from build123d import *

# Parameters (mm, degrees)
BOSS_EXTRUDE1_DEPTH     = 63.5
CUT_EXTRUDE1_DEPTH      = 157.189348228
CUT_EXTRUDE1_DEPTH_BACK = 38.1
CUT_EXTRUDE2_DEPTH      = 157.189348228
CUT_EXTRUDE3_DEPTH      = 180.268046511
SKETCH5_R               = 31.75
CUT_EXTRUDE4_DEPTH      = 19.05
SKETCH6_R               = 9.525
CUT_EXTRUDE5_DEPTH      = 157.189348228
SKETCH7_R               = 15.875
CUT_EXTRUDE6_DEPTH      = 148.69723254


with BuildPart() as part:
    # Sketch1 → Boss-Extrude1 (new body)
    with BuildSketch(Plane(origin=(0, 0, 0), x_dir=(1, 0, 0), z_dir=(0, 1, 0))):
        with BuildLine():
            Line((0, -50.8), (-133.35, -50.8))
            Line((-133.35, -50.8), (-133.35, 50.8))
            Line((-133.35, 50.8), (0, 50.8))
            ThreePointArc((0, 50.8), (50.8, 0), (0, -50.8))
        make_face()
    extrude(amount=BOSS_EXTRUDE1_DEPTH)

    # Sketch2 → Cut-Extrude1 (cut, two sides: drawn at the far end of the back side and taken through both)
    with BuildSketch(Plane(origin=(0, 63.5, 0), x_dir=(1, 0, 0), z_dir=(0, 1, 0)).offset(-CUT_EXTRUDE1_DEPTH_BACK)):
        Polygon((-31.75, 348.168195874), (-31.75, 50.8), (-31.75, -50.8), (-31.75, -348.168195874), (562.986391748, -348.168195874), (562.986391748, 348.168195874), align=None)
    extrude(amount=CUT_EXTRUDE1_DEPTH + CUT_EXTRUDE1_DEPTH_BACK, mode=Mode.SUBTRACT)

    # Sketch3 → Cut-Extrude2 (cut, through all)
    with BuildSketch(Plane(origin=(0, 63.5, 0), x_dir=(1, 0, 0), z_dir=(0, 1, 0))):
        Polygon((-133.35, -50.8), (-50.8, -50.8), (-133.35, -3.139735278), align=None)
    extrude(amount=-CUT_EXTRUDE2_DEPTH, mode=Mode.SUBTRACT)

    # Sketch4 → Cut-Extrude3 (cut, through all)
    with BuildSketch(Plane(origin=(0, 0, -50.8), x_dir=(-1, 0, 0), z_dir=(0, 0, -1))):
        Polygon((133.35, 63.5), (107.95, 63.5), (133.35, 38.1), align=None)
    extrude(amount=-CUT_EXTRUDE3_DEPTH, mode=Mode.SUBTRACT)

    # Sketch5 → Cut-Extrude4 (cut)
    with BuildSketch(Plane(origin=(0, 63.5, 0), x_dir=(1, 0, 0), z_dir=(0, 1, 0))):
        with Locations((-31.75, 0)):
            Circle(SKETCH5_R)
    extrude(amount=-CUT_EXTRUDE4_DEPTH, mode=Mode.SUBTRACT)

    # Sketch6 → Cut-Extrude5 (cut, through all)
    with BuildSketch(Plane(origin=(0, 63.5, 0), x_dir=(1, 0, 0), z_dir=(0, 1, 0))):
        with Locations(Location((-82.55, 25.4, 0), (0, 0, 270))):
            Circle(SKETCH6_R)
    extrude(amount=-CUT_EXTRUDE5_DEPTH, mode=Mode.SUBTRACT)

    # Sketch7 → Cut-Extrude6 (cut, through all)
    with BuildSketch(Plane(origin=(0, 25.4, 0), x_dir=(1, 0, 0), z_dir=(0, 1, 0))):
        with Locations(Location((0, 0, 0), (0, 0, 270))):
            Circle(SKETCH7_R)
    extrude(amount=-CUT_EXTRUDE6_DEPTH, mode=Mode.SUBTRACT)


solid = part.part
Part model, mm, in its own coordinate system. A direction names the side the tool comes from. Give positions to 0.01 mm unless a question says otherwise; leave off trailing zeros. Loops run counter-clockwise (first coordinate to the right, second up) from the corner with the lowest first, then second, coordinate; pieces in that order, holes last. Notation, with made-up numbers: (4.25, 40.25) -> (46.25, 40.25) arc R5 cw to (46.25, 46.25) -> close; hole circle Ø1 at (47.25, 37.25). An arc over 180 degrees is marked (long way). Write each question's results on one line, items separated by ' | '. Start each with the question number.
Q1. Wall check: L1, parallel to X at y = 8, z = 0 (3 decimals); L2, parallel to Y at x = -26.5, z = 26.5; L3, parallel to X at y = 5.5, z = -9.5. Give the ranges that are in metal, low to high.
Q2. Pull direction Z, two halves, no side cores. Call faces 1 (the face through (-91.5, 32.2, 27.3)), 2 (the face through (-15.497, 12.878, -3.441)), 3 (the face through (18, 25.4, -1)), 4 (the face through (-63.492, 54.108, -0.698)): +Z half, -Z half, draft (parallel to the pull), parting line (faces both ways), or undercut.
Q3. Band-saw the part on C-C on y = 35. List the corners of the cut face in (x, z) (3 decimals).
Q4. Band-saw the part on D-D on x = -82.55. List the corners of the cut face in (y, z) (3 decimals).
Q5. Band-saw the part on B-B on y = 22. List the corners of the cut face in (x, z) (3 decimals).
Q6. Pin check, flat tips, straight feed: P1, Ø25, axis at x = 29.5, z = 15, coming from the +Y side; P2, Ø10, axis at y = 9, z = 40.5, coming from the +X side; P3, Ø1, axis at x = 30.5, y = 21, coming from the +Z side; P4, Ø10, axis at x = -87.5, z = -39.5, coming from the -Y side. Stop position of each tip, or through.
Q7. Band-saw the part on A-A on z = 0. List the corners of the cut face in (x, y) (3 decimals).
Q8. Which spindle directions (+Z, -Z, +X, -X, +Y, -Y) get a long thin tool onto all of the face, cutting with end or side? Do faces 5 (the face through (-44, 44.45, 0)), 6 (the face through (-31.75, 40, -1)), 7 (the face through (-69, 63.5, -12)). Say none if no direction does.
Results are:
1) L1: x = -133.35 to -15.875, 15.875 to 50.8 | L2: y = 0 to 25.4 | L3: x = -133.35 to -12.72, 12.72 to 49.9
2) face 1: +Z half | face 2: undercut | face 3: draft | face 4: undercut
3) outline: (-133.35, -50.8) -> (-31.75, -50.8) -> (-31.75, 50.8) -> (-50.8, 50.8) -> (-133.35, 3.14) -> close; hole circle Ø19.05 at (-82.55, -25.4)
4) outline: (0, -50.8) -> (63.5, -50.8) -> (63.5, -34.925) -> (0, -34.925) -> close; (0, -15.875) -> (63.5, -15.875) -> (63.5, 32.469) -> (0, 32.469) -> close
5) outline: (-133.35, -50.8) -> (0, -50.8) arc R50.8 ccw to (0, 50.8) -> (-50.8, 50.8) -> (-133.35, 3.14) -> close; hole circle Ø19.05 at (-82.55, -25.4); hole circle Ø31.75 at (0, 0)
6) P1: stops at y = 25.4 | P2: stops at x = 36.34 | P3: stops at z = 41 | P4: stops at y = 0
7) outline: (-133.35, 0) -> (-15.875, 0) -> (-15.875, 25.4) -> (-31.75, 25.4) -> (-31.75, 44.45) -> (-63.5, 44.45) -> (-63.5, 63.5) -> (-107.95, 63.5) -> (-133.35, 38.1) -> close; (15.875, 0) -> (50.8, 0) -> (50.8, 25.4) -> (15.875, 25.4) -> close
8) face 5: +X, +Y | face 6: +Z, -Z, +X, +Y | face 7: +Z, -Z, +X, -X, +Y
